Geometry check sheet. Reference: the model listing, model coordinates, mm. A direction names the side the tool comes from. Coordinates: 2 decimals unless noted, no trailing zeros. Write each loop counter-clockwise with the first axis right and the second up, starting at its lowest first coordinate (ties: lowest second). Pieces come first, ordered by that corner, then holes. Notation, with made-up numbers: M 34.25,50 L 93.25,50 A19 cw 93.25,56 Z; hole C -10.75,49 d10. An arc over 180 degrees is marked long. Put each result on its own line as item: value. Start each with the question number.
1) Cross-section at D-D on y = 14.75. Record the cut outline in (x, z).
2) Scan lines: line 1 along X through (y, z) = (7.75, 3.75); line 2 along Z through (x, y) = (8.35, 5.1); line 3 along X through (y, z) = (22.75, 1). Record each from-to range of solid material in increasing order.
3) Set-up check for faces 4 (the flat face through (6, 14.1, 1)), 5 (the flat face through (0.99, 7.47, 5.87)), 6 (the flat face through (12, 10.1, 1)), 7 (the flat face through (10.01, 7.47, 5.87)): record each of +Z, -Z, +X, -X, +Y, -Y from which the full face is reachable in a straight line by a thin tool's end or side.
4) Cross-section at A-A on y = 5.1. Record the cut outline in (x, z), plus the area to 3 significant figures.
5) Cross-section at B-B on z = 3.75. Record the cut outline in (x, y).
6) Mould release check, pull along Y, two halves, no side actions. Record for faces 1 (the flat face through (8, 0, 5)), 2 (the flat face through (0.99, 7.49, 8.62)), 3 (the flat face through (3.85, 5, 5)): released by +Y, released by -Y, zero draft, split by the parting line, or undercut.
7) Cross-section at C-C on x = 3. Record the cut outline in (y, z).
8) Gauge pin test, flat ends, axial feed: pin 1 (0.6 mm diameter, centred on x = 9.5, y = 4.5, fed in from -Z); pin 2 (6 mm diameter, centred on y = 6.5, z = 6, fed in from +X); pin 3 (3 mm diameter, centred on x = 2.5, z = 7.5, fed in from +Y); pin 4 (7 mm diameter, centred on x = 7, y = 16.5, fed in from +Z). Record the tip position at first contact, or that the pin passes through.
from build123d import *

# Parameters (mm, degrees)
BOSS_EXTRUDE1_DEPTH = 3
SKETCH5_W           = 3.85
SKETCH5_H           = 10.1
BOSS_EXTRUDE3_DEPTH = 8
CUT_EXTRUDE4_REACH  = 31.357
SKETCH6_R           = 1.6
SKETCH6_3_R         = 1.6
CUT_EXTRUDE5_DEPTH  = 2


with BuildPart() as part:
    # Sketch1 → Boss-Extrude1 (new body)
    with BuildSketch(Plane.XY):
        Polygon((0, 10), (0, 0), (11, 0), (11, 10), (11, 10.1), (12.65, 10.1), (12.65, 24.1), (8.65, 24.1), (8.65, 14.1), (2.35, 14.1), (2.35, 24.1), (-1.65, 24.1), (-1.65, 10.1), (0, 10.1), align=None)
    extrude(amount=BOSS_EXTRUDE1_DEPTH)

    # Sketch5 → Boss-Extrude3 (add)
    with BuildSketch(Plane.XY.offset(3)):
        with Locations((9.075, 5.05)):
            Rectangle(SKETCH5_W, SKETCH5_H)
        with Locations((1.925, 5.05)):
            Rectangle(SKETCH5_W, SKETCH5_H)
    extrude(amount=BOSS_EXTRUDE3_DEPTH)

    # Sketch6 → Cut-Extrude4 (cut, up to next)
    with BuildSketch(Plane(origin=(11, 0, 0), x_dir=(0, 0, -1), z_dir=(1, 0, 0)), mode=Mode.PRIVATE) as cut_extrude4_sk1:
        with Locations(Location((-7.263468762, 5.1, 0), (0, 0, 90))):
            Circle(SKETCH6_R)
    cut_extrude4_tool1 = extrude(cut_extrude4_sk1.sketch, amount=-CUT_EXTRUDE4_REACH, mode=Mode.PRIVATE) & part.part
    cut_extrude4 = cut_extrude4_tool1.solids().sort_by_distance((11, 5.1, 7.263469))[0]
    add(cut_extrude4, mode=Mode.SUBTRACT)

    # Sketch6_3 → Cut-Extrude5 (cut)
    with BuildSketch(Plane(origin=(11, 0, 0), x_dir=(0, 0, -1), z_dir=(1, 0, 0))):
        Polygon((-7.263468762, 8.275426481), (-10.013468762, 6.68771324), (-10.013468762, 3.51228676), (-7.263468762, 1.924573519), (-4.513468762, 3.51228676), (-4.513468762, 6.68771324), align=None)
        with Locations(Location((-7.263468762, 5.1, 0), (0, 0, 90))):
            Circle(SKETCH6_3_R, mode=Mode.SUBTRACT)
    cut_extrude5 = extrude(amount=-CUT_EXTRUDE5_DEPTH, mode=Mode.SUBTRACT)

    # Mirror2: Cut-Extrude4, Cut-Extrude5 across plane
    add(cut_extrude4.mirror(Plane(origin=(5.5, 0, 0), x_dir=(0, 0, 1), z_dir=(1, 0, 0))), mode=Mode.SUBTRACT)
    add(cut_extrude5.mirror(Plane(origin=(5.5, 0, 0), x_dir=(0, 0, 1), z_dir=(1, 0, 0))), mode=Mode.SUBTRACT)


solid = part.part
Answer key:
1. outline: M -1.65,0 L 2.35,0 L 2.35,3 L -1.65,3 Z; M 8.65,0 L 12.65,0 L 12.65,3 L 8.65,3 Z
2. line 1: x = 0 to 3.85, 7.15 to 11
2. line 2: z = 0 to 5.66, 8.86 to 11
2. line 3: x = -1.65 to 2.35, 8.65 to 12.65
3. face 4: +Z, -Z, +Y
3. face 5: -X
3. face 6: +Z, -Z, +X, -Y
3. face 7: +X
4. outline: M 0,0 L 11,0 L 11,4.51 L 9,4.51 L 9,5.66 L 7.15,5.66 L 7.15,3 L 3.85,3 L 3.85,5.66 L 2,5.66 L 2,4.51 L 0,4.51 Z; M 0,10.01 L 2,10.01 L 2,8.86 L 3.85,8.86 L 3.85,11 L 0,11 Z; M 7.15,8.86 L 9,8.86 L 9,10.01 L 11,10.01 L 11,11 L 7.15,11 Z
4. area: 60.8 mm²
5. outline: M 0,0 L 3.85,0 L 3.85,10.1 L 0,10.1 Z; M 7.15,0 L 11,0 L 11,10.1 L 7.15,10.1 Z
6. face 1: released by -Y
6. face 2: undercut
6. face 3: zero draft
7. outline: M 0,0 L 14.1,0 L 14.1,3 L 10.1,3 L 10.1,11 L 0,11 Z; hole C 5.1,7.26 d3.2
8. pin 1: stops at z = 0
8. pin 2: stops at x = 11
8. pin 3: stops at y = 10.1
8. pin 4: stops at z = 3
